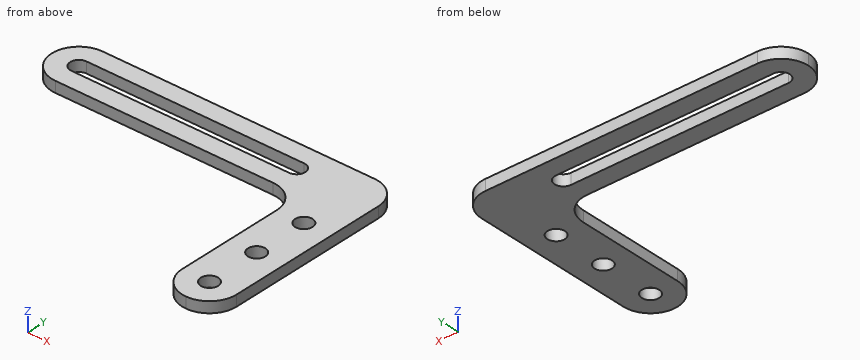
Autodesk Inventor part; units mm, degrees
ref_plane "YZ Plane" through (0, 0, 0) normal (1, 0, 0) x (0, 1, 0)
ref_plane "XZ Plane" through (0, 0, 0) normal (0, 1, 0) x (-1, 0, 0)
ref_plane "XY Plane" through (0, 0, 0) normal (0, 0, 1) x (1, 0, 0)
sketch "スケッチ1" plane through (0, 0, 0) normal (0, 0, 1) x (1, 0, 0)
  line L0 (0, 0) -> (-10, 0)
  line L1 (-10, 0) -> (-10, -30)
  line L2 (-10, -30) -> (0, -30)
  line L3 (0, -30) -> (0, 0)
  line L4 (0, 0) -> (-60, 0)
  line L5 (-60, 0) -> (-60, 10)
  line L6 (-60, 10) -> (0, 10)
  line L7 (0, 10) -> (0, 0)
  line L8 (-5, -30) -> (-5, 0)
  line L9 (0, 5) -> (-60, 5)
  circle A0 centre (-5, 5) radius 1.6
  circle A1 centre (-5, -5) radius 1.6
  circle A2 centre (-15, 5) radius 1.6
  circle A3 centre (-25, 5) radius 1.6
  circle A4 centre (-5, -15) radius 1.6
  circle A5 centre (-35, 5) radius 1.6
  circle A6 centre (-45, 5) radius 1.6
  circle A7 centre (-55, 5) radius 1.6
  line L10 (-5, 3.4) -> (-55, 3.4)
  line L11 (-55, 6.6) -> (-5, 6.6)
  circle A8 centre (-5, -25) radius 1.6
  point P0 (-45, 3.4)
  point P1 (-45, 6.6)
  point P2 (-15, 3.4)
  point P3 (-15, 6.6)
  dimension "d0" = 10
  dimension "d1" = 30
  dimension "d2" = 60
  dimension "d3" = 10
  dimension "d4" = 3.2
  dimension "d5" = 3.2
  dimension "d6" = 5
  dimension "d7" = 5
  dimension "d8" = 10
  dimension "d11" = 10
  dimension "d18" = 10
extrude "押し出し1" add sketch "スケッチ1" along normal blind 2 contours L3 L2 L8 A8 A4 A1 L0 | L0 L4 L5 L9 A7 L10 A0 L7 | L8 A1 A4 A8 L2 L1 L0 | L9 A0 L11 A7 L5 L6 L7 | A0 L9 | L9 A0 | A0 L10 A2 L9 | L9 A2 L11 A0
fillet "フィレット1" radius 5 6 edges at (0, 10, 1) (-60, 10, 1) (-60, 0, 1) (0, -30, 1) (-10, -30, 1) (-10, 0, 1)
properties part number "kakutome_nc_slit"
The listing builds one solid part. Answer for the finished solid, in the listing's coordinates (mm). Give positions to 0.01 mm unless a question says otherwise; leave off trailing zeros. Write each loop counter-clockwise with the first axis right and the second up, starting at its lowest first coordinate (ties: lowest second). Pieces come first, ordered by that corner, then holes. Notation, with made-up numbers: (50, -31.75) -> (64, -31.75) arc R30 ccw to (64, -7.75) -> close; hole circle Ø5 at (63, 30.25). An arc over 180 degrees is marked (long way). One line per question, with ' | ' between items. Start each with the question number.
1. Section B-B (y = -15) is taken. Determine the outline of the cut face in (x, z), plus the area to 3 significant figures.
2. Section A-A (x = -34) is taken. Determine the outline of the cut face in (y, z).
3. Find the intervals of material crossed by probe 1 along Y at (x, z) = (-5, 1.3); probe 2 along X at (y, z) = (-25, 1); probe 3 along Y at (x, z) = (-24.5, 1), in increasing order.
4. Section C-C (z = 0.5) is taken. State how many separate pieces and enclosed holes the cut face has, plus the area to 3 significant figures.
5. Section D-D (x = -11.5) is taken. Determine the outline of the cut face in (y, z), plus the area to 3 significant figures.
6. Given pin 1 Ø0.6 at (x, z) = (-35.5, 1) entering from -Y; pin 2 Ø0.6 at (y, z) = (-16.5, 0.5) entering from -X, each flat-ended and moving along its own axis, determine where each tip first touches the part or whether it passes through.
Response values:
1) outline: (-10, 0) -> (-6.6, 0) -> (-6.6, 2) -> (-10, 2) -> close; (-3.4, 0) -> (0, 0) -> (0, 2) -> (-3.4, 2) -> close | area: 13.6 mm2
2) outline: (0, 0) -> (3.4, 0) -> (3.4, 2) -> (0, 2) -> close; (6.6, 0) -> (10, 0) -> (10, 2) -> (6.6, 2) -> close
3) probe 1: -30 to -26.6, -23.4 to -16.6, -13.4 to -6.6, -3.4 to 10 | probe 2: -10 to -6.6, -3.4 to 0 | probe 3: 0 to 3.4, 6.6 to 10
4) separate pieces: 1 | enclosed holes: 4 | area: 718 mm2
5) outline: (-1.43, 0) -> (10, 0) -> (10, 2) -> (-1.43, 2) -> close | area: 22.9 mm2
6) pin 1: y = 0 | pin 2: x = -10
